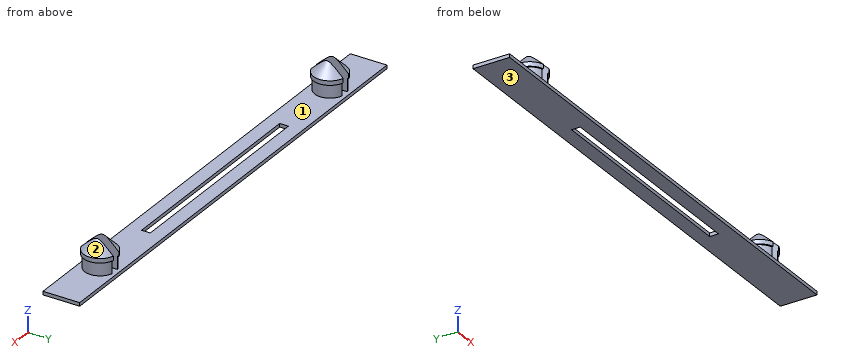
```python
from build123d import *

# Parameters (mm, degrees)
SKICA2_W                 = 55.6
SKICA2_H                 = 4.2
SKICA2_W_2               = 25
SKICA2_H_2               = 1
P_IDAT_VYSUNUT_M2_DEPTH  = 0.4
SKICA3_R                 = 1.75
P_IDAT_VYSUNUT_M3_DEPTH  = 1.5
SKICA5_R                 = 1.9
P_IDAT_VYSUNUT_M5_DEPTH  = 2
ZKOSEN_2_SIZE            = 1.5
SKICA7_W                 = 1
SKICA7_H                 = 5
ODEBRAT_VYSUNUT_M1_DEPTH = 3.5


with BuildPart() as part:
    # Skica2 → Přidat vysunutím2 (new body)
    with BuildSketch(Plane.XY):
        Rectangle(SKICA2_W, SKICA2_H)
        Rectangle(SKICA2_W_2, SKICA2_H_2, mode=Mode.SUBTRACT)
    extrude(amount=P_IDAT_VYSUNUT_M2_DEPTH)

    # Skica3 → Přidat vysunutím3 (add)
    with BuildSketch(Plane.XY.offset(0.4)):
        with Locations((-20.8, 0)):
            Circle(SKICA3_R)
        with Locations((20.8, 0)):
            Circle(SKICA3_R)
    extrude(amount=P_IDAT_VYSUNUT_M3_DEPTH)

    # Skica5 → Přidat vysunutím5 (add)
    with BuildSketch(Plane.XY.offset(1.9)):
        with Locations((-20.8, 0)):
            Circle(SKICA5_R)
        with Locations((20.8, 0)):
            Circle(SKICA5_R)
    extrude(amount=P_IDAT_VYSUNUT_M5_DEPTH)

    # Zkosení2
    zkosen_2_edges = [part.edges().sort_by_distance(p)[0] for p in [
        (-22.7, 0, 3.9),
        (18.9, 0, 3.9),
    ]]
    chamfer(zkosen_2_edges, length=ZKOSEN_2_SIZE)

    # Skica7 → Odebrat vysunutím1 (cut)
    with BuildSketch(Plane.XY.offset(3.9)):
        with Locations((-20.8, 0)):
            Rectangle(SKICA7_W, SKICA7_H)
        with Locations((20.8, 0)):
            Rectangle(SKICA7_W, SKICA7_H)
    extrude(amount=-ODEBRAT_VYSUNUT_M1_DEPTH, mode=Mode.SUBTRACT)


solid = part.part
```
Geometry check sheet. Reference: the model listing, model coordinates, mm. Face numbers are marked on the shaded views. Coordinates: 2 decimals unless noted, no trailing zeros. Loops run counter-clockwise (first coordinate to the right, second up) from the corner with the lowest first, then second, coordinate; pieces in that order, holes last. Notation, with made-up numbers: (32.5, 73.5) - (65.5, 73.5) arc R21 ccw to (65.5, 106.5) - close; hole circle Ø2 at (20.25, 35.5). An arc over 180 degrees is marked (long way). One line per item, written item: value. Start each with the question number.
(1) Mould release check, pull along X, two halves, no side actions. Record for the marked faces 1, 2 and 3: released by +X, released by -X, zero draft, split by the parting line, or undercut.
(2) Cross-section at A-A on x = 5. Enter the section's corners in (y, z).
(3) Material ranges on line 1 (X direction, y = 0.2, z = 1.5); line 2 (X direction, y = 0.6, z = 3.25); line 3 (X direction, y = 0.4, z = 0.3), recorded low to high. Write a range as [from, to].
(4) Cross-section at B-B on z = 1.35. Enter the section's corners in (x, y).
(5) Depth check by flat-ended pin: P1, Ø1.5, axis at x = 10.5, y = -0.5, coming from the +Z side; P2, Ø1, axis at y = 0, z = 2.5, coming from the +X side; P3, Ø1, axis at x = -12, z = 1, coming from the -Y side; P4, Ø2, axis at x = -3, y = 1, coming from the -Z side. Enter the tip coordinate at first touch or a pass-through.
Results below:
1. face 1: undercut
1. face 2: released by +X
1. face 3: zero draft
2. outline: (-2.1, 0) - (-0.5, 0) - (-0.5, 0.4) - (-2.1, 0.4) - close; (0.5, 0) - (2.1, 0) - (2.1, 0.4) - (0.5, 0.4) - close
3. line 1: x = [-22.54, -21.3], [-20.3, -19.06], [19.06, 20.3], [21.3, 22.54]
3. line 2: x = [-21.66, -21.3], [-20.3, -19.94], [19.94, 20.3], [21.3, 21.66]
3. line 3: x = [-27.8, -12.5], [12.5, 27.8]
4. outline: (-21.3, -1.68) - (-21.3, 1.68) arc R1.75 ccw to start; (-20.3, -1.68) arc R1.75 ccw to (-20.3, 1.68) - close; (20.3, -1.68) - (20.3, 1.68) arc R1.75 ccw to start; (21.3, -1.68) arc R1.75 ccw to (21.3, 1.68) - close
5. P1: stops at z = 0.4
5. P2: stops at x = 22.7
5. P3: passes through
5. P4: stops at z = 0
